Study the drawing (mm; zero at the part's minimum x, y, z) and answer. Give positions to 0.01 mm unless a question says otherwise; leave off trailing zeros. Order: outer loops, then holes, each group sorted by start corner. A loop starts at its lowest first (then second) coordinate and runs counter-clockwise, first axis right, second up. Notation, with made-up numbers: (62.25, 63.25) - (82.25, 63.25) arc R25 ccw to (82.25, 93.25) - close; hole circle Ø11 at (85, 77.5). An arc over 180 degrees is marked (long way). Return JSON: item names as keys, results as strings.
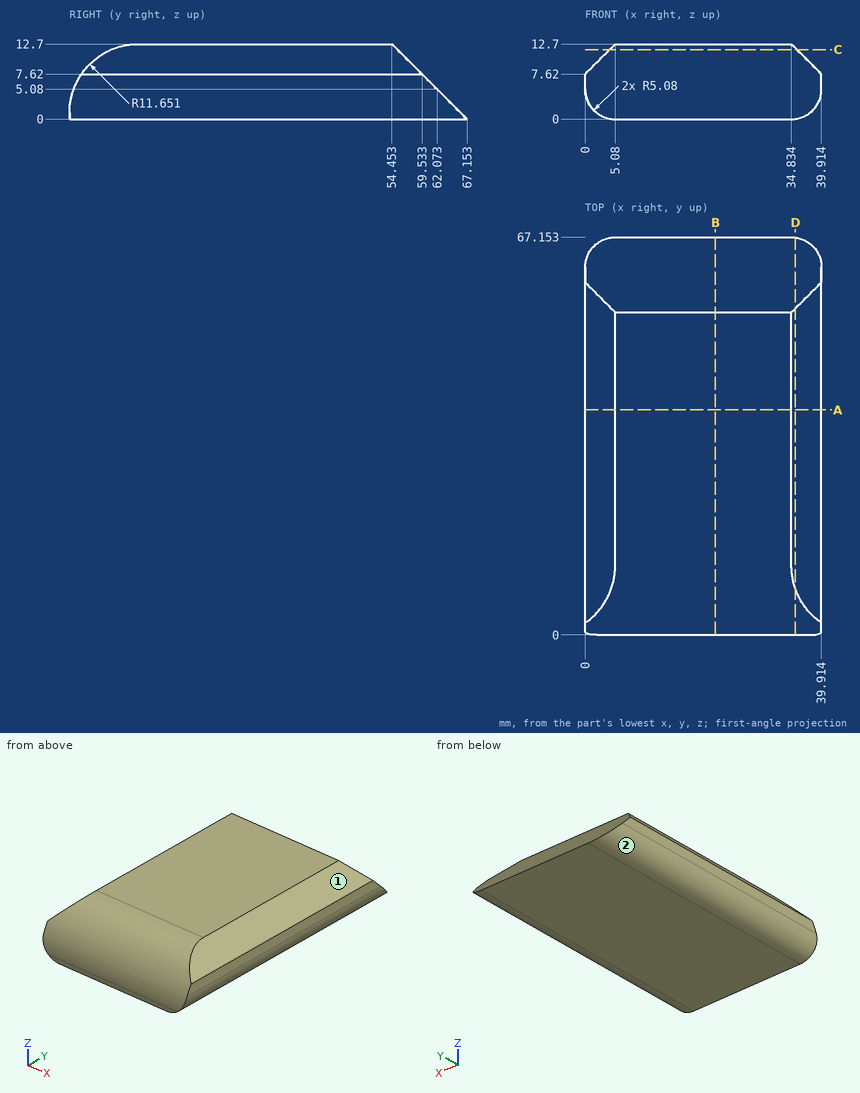
Q1. A cutting plane is placed at A-A (y = 38). Write down the section's boundary in (x, z).
Values:
{"outline": "(0, 5.08) arc R5.08 ccw to (5.08, 0) - (34.83, 0) arc R5.08 ccw to (39.91, 5.08) - (39.91, 7.62) - (34.83, 12.7) - (5.08, 12.7) - (0, 7.62) - close"}
Q2. A cutting plane is placed at D-D (x = 35.5). Write down the section's boundary in (y, z).
Values:
{"outline": "(0, 0.04) - (67.11, 0.04) - (55.12, 12.03) - (7.77, 12.03) arc R11.65 ccw to (0, 1.05) - close"}
Q3. A cutting plane is placed at C-C (z = 11.75). Write down the section's boundary in (x, y), and give its area (3 significant figures).
Values:
{"outline": "(4.13, 7.04) - (35.78, 7.04) - (35.78, 55.4) - (4.13, 55.4) - close", "area": "1,530 mm²"}
Q4. A cutting plane is placed at B-B (x = 22). Write down the section's boundary in (y, z).
Values:
{"outline": "(0, 0) - (67.15, 0) - (54.45, 12.7) - (11.65, 12.7) arc R11.65 ccw to (0, 1.05) - close"}
Q5. Determine the mould class of the marked faces 1 and 2 for opening direction Z: released by +Z, released by -Z, zero draft, split by the parting line, or undercut.
Values:
{"face 1": "released by +Z", "face 2": "released by -Z"}
Q6. Consider L1, parallel to Y at x = 7, z = 1; L2, parallel to X at y = 24.5, z = 4; L3, parallel to Y at x = 11, z = 5.25. Determine where each line is inside the solid, lowest interval first.
Values:
{"L1": "y = 0 to 66.15", "L2": "x = 0.12 to 39.8", "L3": "y = 0.78 to 61.9"}
Q7. Given pin 1 (2 mm diameter, centred on x = 31.5, z = 3, fed in from +Y); pin 2 (1.5 mm diameter, centred on x = 23.5, z = 2.5, fed in from -Y); pin 3 (2 mm diameter, centred on x = 31, z = 9, fed in from +Y), each flat-ended and moving along its own axis, determine where each tip first touches the part or whether it passes through.
Values:
{"pin 1": "stops at y = 65.15", "pin 2": "stops at y = 0.02", "pin 3": "stops at y = 59.15"}
